Model file for the job. Use its own axes, mm. Round coordinates to 2 decimals unless told otherwise and drop trailing zeros. Write each loop counter-clockwise with the first axis right and the second up, starting at its lowest first coordinate (ties: lowest second). Pieces come first, ordered by that corner, then holes. Notation, with made-up numbers: (4, 21.5) - (58, 21.5) arc R28 ccw to (58, 45.5) - close; hole circle Ø7 at (6.25, 83.5). An arc over 180 degrees is marked (long way). Answer as a JSON object with one key per item and string values. Group by question number.
from build123d import *

# Parameters (mm, degrees)
SKETCH1_R             = 87.5
BOSS_EXTRUDE1_DEPTH   = 10
SKETCH2_R             = 7.5
CUT_EXTRUDE1_DEPTH    = 125.147090179
SKETCH3_R             = 3.721577815
CUT_EXTRUDE2_DEPTH    = 8.414034
CIRPATTERN1_START     = 1.585966326
CIRPATTERN1_OUTLINE_R = 3.721577815
CIRPATTERN1_DEPTH     = 8.414033674


# Read off the part's stored shape, not the designer's step: CirPattern1
with BuildPart() as part:
    # Sketch1 → Boss-Extrude1 (new body)
    with BuildSketch(Plane(origin=(0, 0, 0), x_dir=(1, 0, 0), z_dir=(0, 1, 0))):
        with Locations(Location((0, 0, 0), (0, 0, 270))):
            Circle(SKETCH1_R)
    extrude(amount=BOSS_EXTRUDE1_DEPTH)

    # Sketch2 → Cut-Extrude1 (cut, through all)
    with BuildSketch(Plane(origin=(0, 0, 0), x_dir=(1, 0, 0), z_dir=(0, 1, 0))):
        with Locations(Location((0, 0, 0), (0, 0, 270))):
            Circle(SKETCH2_R)
    extrude(amount=CUT_EXTRUDE1_DEPTH, mode=Mode.SUBTRACT)

    # Sketch3 → Cut-Extrude2 (cut)
    with BuildSketch(Plane(origin=(0, 10, 0), x_dir=(1, 0, 0), z_dir=(0, 1, 0))):
        with Locations(Location((-40.642213715, 0, 0), (0, 0, 270))):
            Circle(SKETCH3_R)
    extrude(amount=-CUT_EXTRUDE2_DEPTH, mode=Mode.SUBTRACT)

    # CirPattern1 outline → CirPattern1 (cut)
    with BuildSketch(Plane(origin=(0, 0, 0), x_dir=(1, 0, 0), z_dir=(0, 1, 0)).offset(CIRPATTERN1_START)):
        with Locations((-12.559134727, 38.653042191)):
            Circle(CIRPATTERN1_OUTLINE_R)
        with Locations((32.880241585, 23.888893842)):
            Circle(CIRPATTERN1_OUTLINE_R)
        with Locations((32.880241585, -23.888893842)):
            Circle(CIRPATTERN1_OUTLINE_R)
        with Locations((-12.559134727, -38.653042191)):
            Circle(CIRPATTERN1_OUTLINE_R)
    extrude(amount=CIRPATTERN1_DEPTH, mode=Mode.SUBTRACT)


solid = part.part
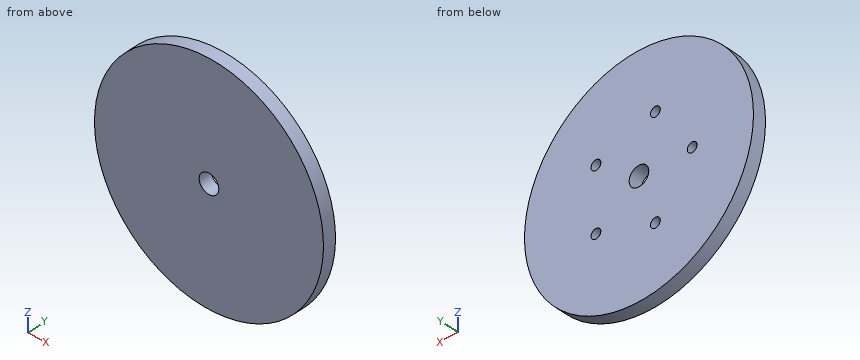
(1) Slice it at D-D (x = 74.5). Write the cut outline in (y, z), then the cut area to 3 significant figures.
(2) Slice it at C-C (y = 8.25). Write the cut outline in (x, z), then the cut area to 3 significant figures.
(3) Slice it at A-A (z = 0). Write the cut outline in (x, y).
(4) Drill centre lines: line 1 (X direction, y = 5, z = 0); line 2 (X direction, y = 3.75, z = 3); line 3 (Z direction, x = 30, y = 7.5). Where is each one in solid material? Low to high. Write a range as from..to.
(5) Slice it at B-B (x = 0). Write the cut outline in (y, z), then the cut area to 3 significant figures.
(6) Flat gauge pins, fed straight in: pin 1 (5 mm diameter, centred on y = 3, z = -12, fed in from -X); pin 2 (2 mm diameter, centred on x = 31, z = -22, fed in from +Y); pin 3 (12 mm diameter, centred on x = 0, z = 0, fed in from +Y); pin 4 (1 mm diameter, centred on x = 69, y = 4.5, fed in from +Z). Where does each tip first touch, or does it go through?
Answer:
{
 "1": {"outline": "(0, -45.89) - (10, -45.89) - (10, 45.89) - (0, 45.89) - close", "area": "918 mm²"},
 "2": {"outline": "circle Ø175 at (0, 0); hole circle Ø7.44 at (-40.64, 0); hole circle Ø7.44 at (-12.56, -38.65); hole circle Ø7.44 at (-12.56, 38.65); hole circle Ø15 at (0, 0); hole circle Ø7.44 at (32.88, -23.89); hole circle Ø7.44 at (32.88, 23.89)", "area": "23,700 mm²"},
 "3": {"outline": "(-87.5, 0) - (-7.5, 0) - (-7.5, 10) - (-36.92, 10) - (-36.92, 1.59) - (-44.36, 1.59) - (-44.36, 10) - (-87.5, 10) - close; (7.5, 0) - (87.5, 0) - (87.5, 10) - (7.5, 10) - close"},
 "4": {"line 1": "-87.5..-44.36, -36.92..-7.5, 7.5..87.5", "line 2": "-87.45..-42.84, -38.44..-6.87, 6.87..87.45", "line 3": "-82.2..-26.25, -21.53..21.53, 26.25..82.2"},
 "5": {"outline": "(0, -87.5) - (10, -87.5) - (10, -7.5) - (0, -7.5) - close; (0, 7.5) - (10, 7.5) - (10, 87.5) - (0, 87.5) - close", "area": "1,600 mm²"},
 "6": {"pin 1": "x = -86.98", "pin 2": "y = 1.59", "pin 3": "through", "pin 4": "z = 54.44"}
}
